Geometry: final body of the model. Coordinates: model frame, mm. Face numbers are marked on the shaded views. A direction names the side the tool comes from. Give positions to 0.01 mm unless a question says otherwise; leave off trailing zeros. Write each loop counter-clockwise with the first axis right and the second up, starting at its lowest first coordinate (ties: lowest second). Pieces come first, ordered by that corner, then holes.
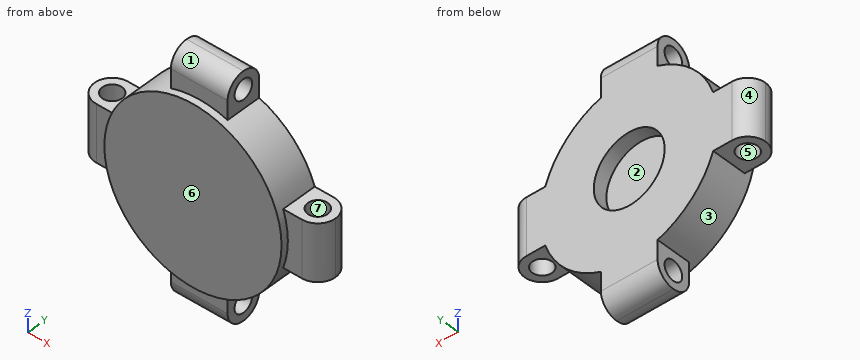
Autodesk Inventor part; units mm, degrees
ref_plane "YZ Plane" through (0, 0, 0) normal (1, 0, 0) x (0, 1, 0)
ref_plane "XZ Plane" through (0, 0, 0) normal (0, 1, 0) x (-1, 0, 0)
ref_plane "XY Plane" through (0, 0, 0) normal (0, 0, 1) x (1, 0, 0)
sketch "Sketch1" plane through (0, 0, 0) normal (0, 1, 0) x (-1, 0, 0)
  circle A0 centre (0, 0) radius 7.9375
  dimension "d0" = 15.875
extrude "Extrusion1" add sketch "Sketch1" along normal blind 3.81
sketch "Sketch2" plane through (0, 3.81, 0) normal (0, 1, 0) x (1, 0, 0)
  circle A0 centre (0, 0) radius 3.175
  dimension "d3" = 6.35
sketch "Sketch3" plane through (0, 0, 0) normal (1, 0, 0) x (0, 1, 0)
  line L0 (0.635, -2.54) -> (3.81, -2.54)
  line L1 (3.81, -2.54) -> (3.81, 2.54)
  line L2 (3.81, 2.54) -> (0.635, 2.54)
  line L3 (3.81, -7.9375) -> (3.81, 7.9375)
  line L4 (0.635, 2.54) -> (0.635, -2.54)
  point P0 (0, 0)
  dimension "d9" = 3.175
  dimension "d20" = 3.175
extrude "Extrusion3" add sketch "Sketch3" along normal mid plane 21.59
fillet "Fillet1" radius 1.5875 4 edges at (10.795, 3.81, 0) (-10.795, 3.81, 0) (10.795, 0.635, 0) (-10.795, 0.635, 0)
sketch "Sketch6" plane through (-7.5201, 0.635, 2.54) normal (0, 0, 1) x (1, 0, 0)
  arc A0 (-1.6874, 3.175) -> (-1.6874, 0) centre (-1.6874, 1.5875) ccw
  circle A1 centre (-1.6874, 1.5875) radius 0.889
  arc A2 (16.7276, 0) -> (16.7276, 3.175) centre (16.7276, 1.5875) ccw
  circle A3 centre (16.7276, 1.5875) radius 0.889
  point P0 (7.5201, -0.635)
  dimension "d25" = 1.778
  dimension "d26" = 1.778
extrude "Extrusion7" cut sketch "Sketch6" against normal through all
pattern_circular "Circular Pattern3" count 2 over 90 about axis through (0, 0, 0) along (0, 1, 0) of "Extrusion3", "Fillet1", "Extrusion7"
extrude "Extrusion8" cut sketch "Sketch2" against normal blind 1.27
properties part number "scrambler_vertical_cap"
Q1. Section D-D on z = 6.25. Output: boundary loops of the cut face in (x, y).
Filled sheet:
outline: (-4.89, 0) - (4.89, 0) - (4.89, 3.81) - (-4.89, 3.81) - close
Q2. Access query for the marked faces 1, 2 and 3. Directions: +Z, -Z, +X, -X, +Y, -Y. A direction counts if a zero-diameter tool reaches every point of the face in a straight line with its end or side. Return the directions, or none.
Filled sheet:
face 1: +Z, +X, -X, -Y
face 2: +Y
face 3: -Y
Q3. Ray query, line 1 along Z through (x, y) = (2, 3); line 2 along Z through (x, y) = (-0.25, 1.5); line 3 along Y through (x, z) = (-9.25, -2.25). Return the intervals inside material, ascending.
Filled sheet:
line 1: z = -10.59 to -9.64, -8.78 to -2.47, 2.47 to 8.78, 9.64 to 10.59
line 2: z = -10.62 to -9.73, -8.69 to 8.69, 9.73 to 10.62
line 3: y = 0.64 to 1.33, 3.11 to 3.81
Q4. Pull-direction query (X, two-part tool) for the marked faces 4, 5, 6 and 7; classes: released by +X, released by -X, zero draft, split by the parting line, or undercut.
Filled sheet:
face 4: released by -X
face 5: undercut
face 6: zero draft
face 7: undercut
Q5. Section A-A on x = 0.75. Count the separate pieces of the cut face and the enclosed holes in it, plus the area to 3 significant figures.
Filled sheet:
separate pieces: 1
enclosed holes: 2
area: 63.6 mm2
Q6. Pin query (flat end, axial travel): P1, Ø2, axis at y = 2.22, z = 9.21, coming from the +X side; P2, Ø2, axis at y = 1, z = -6.5, coming from the +X side; P3, Ø2, axis at y = 2.22, z = -9.21, coming from the -X side. Return the tip coordinate at first contact, or that it passes through.
Filled sheet:
P1: stops at x = 2.54
P2: stops at x = 5.72
P3: stops at x = -2.54
